from build123d import *

# Parameters (mm, degrees)
BOSS_EXTRUDE1_DEPTH = 15
BOSS_EXTRUDE1_DRAFT = -1
SHELL1_T            = -1


with BuildPart() as part:
    # Sketch4 → Boss-Extrude1 (with draft: the straight prism first)
    with BuildSketch(Plane.XY):
        Polygon((134.568658859, 69.541396533), (54.766431957, 69.541396533), (54.766431957, 50.647773961), (54.667545408, 34.886919054), (23.782154036, 5.541396533), (165.55293678, 5.541396533), (134.667545408, 34.886919054), (134.568658859, 50.647773961), align=None)
    extrude(amount=BOSS_EXTRUDE1_DEPTH)
    # Boss-Extrude1: the draft: its side faces are tilted about the plane it starts from
    boss_extrude1_sides = [part.faces().sort_by_distance(p)[0] for p in [
        (94.667545408, 69.541396533, 7.5),
        (54.766431957, 60.094585247, 7.5),
        (54.716988683, 42.767346508, 7.5),
        (39.224849722, 20.214157793, 7.5),
        (94.667545408, 5.541396533, 7.5),
        (150.110241094, 20.214157793, 7.5),
        (134.618102134, 42.767346508, 7.5),
        (134.568658859, 60.094585247, 7.5),
    ]]
    draft(boss_extrude1_sides, Plane.XY, BOSS_EXTRUDE1_DRAFT)

    # Shell1
    shell1_openings = [part.faces().sort_by_distance(p)[0] for p in [
        (94.667545408, 34.129623645, 15),
    ]]
    offset(amount=SHELL1_T, openings=shell1_openings, kind=Kind.INTERSECTION)


solid = part.part
Could you check a few things on this model? Use its own coordinates, in mm. Give positions to 0.01 mm unless a question says otherwise; leave off trailing zeros. Write each loop counter-clockwise with the first axis right and the second up, starting at its lowest first coordinate (ties: lowest second). Pieces come first, ordered by that corner, then holes. Notation, with made-up numbers: (6.25, 21.25) - (53.25, 21.25) arc R26 cw to (53.25, 50.25) - close; hole circle Ø7 at (25.25, 38.25). An arc over 180 degrees is marked (long way). Use CSV: the item, a comma, the result in double quotes. Start each with the question number.
Item 1: I want a section at D-D, the plane z = 13.25. Please give me the cut outline in (x, y), then the cut area to 3 significant figures.
Item 2: If I drill on line 1 along Y through (x, z) = (62.5, 14); line 2 along X through (y, z) = (35.5, 9.5); line 3 along Z through (x, y) = (80.5, 47), over which ranges is the centre line in solid material (lowest first)?
Item 3: I want a section at C-C, the plane y = 30.5. Please give me the cut outline in (x, z).
Item 4: I'm going to push flat-ended pins straight in: pin 1 (6 mm diameter, centred on x = 102, z = 5.5, fed in from -Y); pin 2 (1.5 mm diameter, centred on x = 101.5, y = 46, fed in from +Z); pin 3 (1 mm diameter, centred on x = 78, z = 11, fed in from +Y). Where does each tip first touch, or does it pass through?
Item 5: I want a section at B-B, the plane x = 121. Please give me the cut outline in (y, z), then the cut area to 3 significant figures.
Item 6: I want a section at A-A, the plane z = 2.75. Please give me the cut outline in (x, y), then the cut area to 3 significant figures.
Item 7: If we mould it in two halves opening along X, with no side actions, what happens to faces 1 (the face through (94, 38, 0)), 2 (the face through (94, 38, 1))? For each: pulls with the +X half, pulls with the -X half, needs draft (parallel to the pull), parting line crosses it, or undercut.
Findings:
1,outline,"(23.2, 5.31) - (166.13, 5.31) - (134.9, 34.99) - (134.8, 50.65) - (134.8, 69.77) - (54.54, 69.77) - (54.54, 50.65) - (54.44, 34.99) - close; hole (25.71, 6.31) - (163.63, 6.31) - (133.9, 34.55) - (133.8, 50.65) - (133.8, 68.77) - (55.54, 68.77) - (55.54, 50.65) - (55.43, 34.55) - close"
1,area,"373 mm2"
2,line 1,"y = 5.3 to 6.3, 68.79 to 69.79"
2,line 2,"x = 54.51 to 55.51, 133.83 to 134.83"
2,line 3,"z = 0 to 1"
3,outline,"(49.67, 15) - (50.05, 0) - (139.28, 0) - (139.66, 15) - (138.21, 15) - (137.86, 1) - (51.48, 1) - (51.12, 15) - close"
4,pin 1,"stops at y = 5.39"
4,pin 2,"stops at z = 1"
4,pin 3,"stops at y = 69.74"
5,outline,"(5.28, 15) - (5.54, 0) - (69.54, 0) - (69.8, 15) - (68.8, 15) - (68.56, 1) - (6.52, 1) - (6.28, 15) - close"
5,area,"92.0 mm2"
6,outline,"(23.66, 5.49) - (165.67, 5.49) - (134.72, 34.91) - (134.62, 50.65) - (134.62, 69.59) - (54.72, 69.59) - (54.72, 50.65) - (54.62, 34.91) - close; hole (26.17, 6.49) - (163.17, 6.49) - (133.72, 34.48) - (133.62, 50.64) - (133.62, 68.59) - (55.72, 68.59) - (55.72, 50.64) - (55.62, 34.48) - close"
6,area,"371 mm2"
7,face 1,"needs draft"
7,face 2,"undercut"
